Input: part model. Units: mm. Frame: model coordinates. A direction names the side the tool comes from. Give positions to 0.01 mm unless a question says otherwise; leave off trailing zeros. Write each loop counter-clockwise with the first axis right and the second up, starting at its lowest first coordinate (ties: lowest second). Pieces come first, ordered by that corner, then holes. Notation, with made-up numbers: (-22, 84) - (-13, 84) arc R8 ccw to (-13, 94) - close; hole circle Ø9 at (79.25, 79.5). An arc over 180 degrees is marked (long way). Answer as CSV lines item,"result". Start each with the question number.
from build123d import *

# Parameters (mm, degrees)
SKETCH1_R               = 3
SKETCH1_W               = 3.6
SKETCH1_H               = 3.6
BOSS_EXTRUDE1_DEPTH     = 4
SKETCH2_W               = 3.6
SKETCH2_H               = 3.6
BOSS_EXTRUDE2_DEPTH     = 1
SKETCH3_R               = 3
BOSS_EXTRUDE3_DEPTH     = 1
CUT_EXTRUDE2_DEPTH      = 10.669539803
CUT_EXTRUDE2_DEPTH_BACK = 10.669539803


with BuildPart() as part:
    # Sketch1 → Boss-Extrude1 (new body)
    with BuildSketch(Plane(origin=(0, 0, 0), x_dir=(0, 0, -1), z_dir=(1, 0, 0))):
        Circle(SKETCH1_R)
        Rectangle(SKETCH1_W, SKETCH1_H, mode=Mode.SUBTRACT)
    extrude(amount=BOSS_EXTRUDE1_DEPTH)

    # Sketch2 → Boss-Extrude2 (add)
    with BuildSketch(Plane.ZY):
        with BuildLine():
            Line((-4, 3.5), (4, 3.5))
            ThreePointArc((4, 3.5), (7.5, 0), (4, -3.5))
            Line((4, -3.5), (-4, -3.5))
            ThreePointArc((-4, -3.5), (-7.5, 0), (-4, 3.5))
        make_face()
        Rectangle(SKETCH2_W, SKETCH2_H, mode=Mode.SUBTRACT)
    extrude(amount=-BOSS_EXTRUDE2_DEPTH)

    # Sketch3 → Boss-Extrude3 (add)
    with BuildSketch(Plane(origin=(4, 0, 0), x_dir=(0, 0, -1), z_dir=(1, 0, 0))):
        with Locations(Location((0, 0, 0), (0, 0, 180))):
            Circle(SKETCH3_R)
    extrude(amount=BOSS_EXTRUDE3_DEPTH)

    # Sketch5 → Cut-Extrude2 (cut, two sides: drawn at the far end of the back side and taken through both)
    with BuildSketch(Plane(origin=(0, 0, 0), x_dir=(1, 0, 0), z_dir=(0, 1, 0)).offset(-CUT_EXTRUDE2_DEPTH_BACK)):
        Polygon((5, 2.86), (4.5, 2.36), (5, 1.86), align=None)
        Polygon((5, 1.68), (4.5, 1.18), (5, 0.68), align=None)
        Polygon((5, 0.5), (4.5, 0), (5, -0.5), align=None)
        Polygon((5, -0.68), (4.5, -1.18), (5, -1.68), align=None)
        Polygon((5, -1.86), (4.5, -2.36), (5, -2.86), align=None)
    extrude(amount=CUT_EXTRUDE2_DEPTH + CUT_EXTRUDE2_DEPTH_BACK, mode=Mode.SUBTRACT)


solid = part.part
1) Cut plane C-C on z = 6. Output: boundary loops of the cut face in (x, y), and give its area (3 significant figures).
2) Pull-direction query (Z, two-part tool) for faces 4 (the cylindrical face through (0.5, 0.1, 7.5)), 5 (the flat face through (4, 0, 0)), 6 (the cylindrical face through (0.5, -0.1, -7.5)); classes: +Z half, -Z half, draft (parallel to the pull), parting line (faces both ways), or undercut.
3) Reachability of faces 1 (the cylindrical face through (3, 3, 0)), 2 (the flat face through (0, 2, 0)), 3 (the flat face through (2, 0, 1.8)) from +Z, -Z, +X, -X, +Y, -Y: full face, straight path, thin tool, end or side. Return the list, or none.
4) Contact query for flat-ended pins moving along their axis: P1, Ø3, axis at x = 3.5, z = -2.5, coming from the -Y side; P2, Ø1, axis at y = 0, z = 0.5, coming from the -X side; P3, Ø1.1, axis at x = 2.5, z = 1, coming from the +Y side. Output: stop coordinate, or through.
5) Material intervals for line 1 (X direction, y = 3.25, z = 1.5); line 2 (Y direction, x = 0.65, z = -1.5); line 3 (Z direction, x = 3.7, y = -1.5), sorted ascending. Write a range as from..to.
6) Cut plane A-A on x = 1.8. Output: boundary loops of the cut face in (y, z).
7) Cut plane D-D on z = -5.5. Output: boundary loops of the cut face in (x, y).
8) Cut plane B-B on x = 0.55. Output: boundary loops of the cut face in (y, z), and give its area (3 significant figures).
Numbers:
1,outline,"(0, -2.87) - (1, -2.87) - (1, 2.87) - (0, 2.87) - close"
1,area,"5.74 mm²"
2,face 4,"+Z half"
2,face 5,"undercut"
2,face 6,"-Z half"
3,face 1,"+X"
3,face 2,"+Z, -Z, -X, +Y, -Y"
3,face 3,"-X"
4,P1,"stops at y = -2.83"
4,P2,"stops at x = 4"
4,P3,"stops at y = 2.97"
5,line 1,"x = 0..1"
5,line 2,"y = -3.5..-1.8, 1.8..3.5"
5,line 3,"z = -2.6..-1.8, 1.8..2.6"
6,outline,"circle Ø6 at (0, 0); hole (-1.8, -1.8) - (1.8, -1.8) - (1.8, 1.8) - (-1.8, 1.8) - close"
7,outline,"(0, -3.16) - (1, -3.16) - (1, 3.16) - (0, 3.16) - close"
8,outline,"(-3.5, -4) arc R3.5 ccw to (3.5, -4) - (3.5, 4) arc R3.5 ccw to (-3.5, 4) - close; hole (-1.8, -1.8) - (1.8, -1.8) - (1.8, 1.8) - (-1.8, 1.8) - close"
8,area,"81.5 mm²"
